Geometry check sheet. Reference: drawing and pictorial views, mm from the part's lowest x, y, z. Coordinates: 2 decimals unless noted, no trailing zeros. Order: outer loops, then holes, each group sorted by start corner. A loop starts at its lowest first (then second) coordinate and runs counter-clockwise, first axis right, second up. Notation, with made-up numbers: (-29, 30.5) -> (20, 30.5) arc R16 ccw to (20, 58.5) -> close; hole circle Ø5 at (-23.75, -24). An arc over 180 degrees is marked (long way). Use CSV: the item, a comma, the result in double quotes. Start each with the question number.
1) Sectioned sample at D-D on y = 2.5. Record the boundary of the cut face in (x, z), then the cut area to 3 significant figures.
2) Release check for a two-part mould opening along X. For the marked faces 1, 2 and 3 record: released by +X, released by -X, zero draft, split by the parting line, or undercut.
3) Go/stop test with flat-tipped pins: pin 1 (4 mm diameter, centred on y = 2.5, z = 8, fed in from -X); pin 2 (3 mm diameter, centred on y = 6.5, z = 7, fed in from -X); pin 3 (6 mm diameter, centred on y = 7.5, z = 3.5, fed in from +X). Record where each tip stops, or that it passes through.
4) Scan lines: line 1 along X through (y, z) = (5.5, 5.75); line 2 along X through (y, z) = (2.25, 5.25); line 3 along Y through (x, z) = (9, 0.5). Record each from-to range of solid material in increasing order.
5) Sectioned sample at A-A on y = 8.5. Record the boundary of the cut face in (x, z).
6) Sectioned sample at B-B on z = 6. Record the boundary of the cut face in (x, y) (3 decimals), then the cut area to 3 significant figures.
7) Sectioned sample at C-C on x = 28. Record the boundary of the cut face in (y, z) (3 decimals).
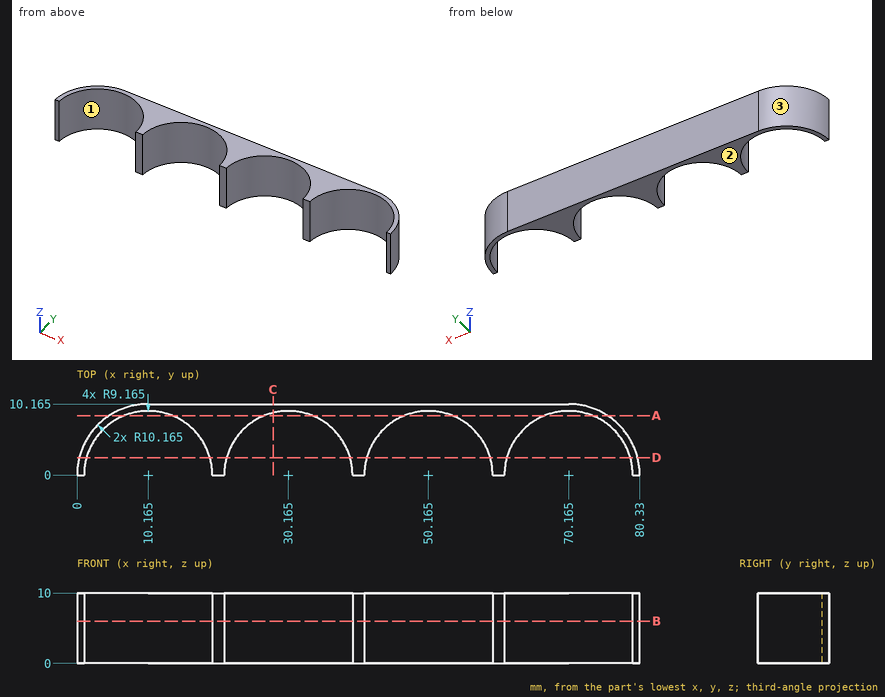
Answers follow:
1,outline,"(0.31, 0) -> (1.35, 0) -> (1.35, 10) -> (0.31, 10) -> close; (18.98, 0) -> (21.35, 0) -> (21.35, 10) -> (18.98, 10) -> close; (38.98, 0) -> (41.35, 0) -> (41.35, 10) -> (38.98, 10) -> close; (58.98, 0) -> (61.35, 0) -> (61.35, 10) -> (58.98, 10) -> close; (78.98, 0) -> (80.02, 0) -> (80.02, 10) -> (78.98, 10) -> close"
1,area,"91.7 mm²"
2,face 1,"undercut"
2,face 2,"zero draft"
2,face 3,"released by -X"
3,pin 1,"stops at x = 0.01"
3,pin 2,"stops at x = 1.31"
3,pin 3,"stops at x = 79.28"
4,line 1,"x = 1.62 to 2.83, 17.5 to 22.83, 37.5 to 42.83, 57.5 to 62.83, 77.5 to 78.71"
4,line 2,"x = 0.25 to 1.28, 19.05 to 21.28, 39.05 to 41.28, 59.05 to 61.28, 79.05 to 80.08"
4,line 3,"y = 9.09 to 10.1"
5,outline,"(4.59, 0) -> (6.74, 0) -> (6.74, 10) -> (4.59, 10) -> close; (13.59, 0) -> (26.74, 0) -> (26.74, 10) -> (13.59, 10) -> close; (33.59, 0) -> (46.74, 0) -> (46.74, 10) -> (33.59, 10) -> close; (53.59, 0) -> (66.74, 0) -> (66.74, 10) -> (53.59, 10) -> close; (73.59, 0) -> (75.74, 0) -> (75.74, 10) -> (73.59, 10) -> close"
6,outline,"(0, 0) -> (1, 0) arc R9.165 cw to (19.33, 0) -> (21, 0) arc R9.165 cw to (39.33, 0) -> (41, 0) arc R9.165 cw to (59.33, 0) -> (61, 0) arc R9.165 cw to (79.33, 0) -> (80.33, 0) arc R10.165 ccw to (70.165, 10.165) -> (10.165, 10.165) arc R10.165 ccw to start"
6,area,"244 mm²"
7,outline,"(8.906, 0) -> (10.165, 0) -> (10.165, 10) -> (8.906, 10) -> close"
